from build123d import *

# Parameters (mm, degrees)
SZKIC2_W                    = 85
SZKIC2_H                    = 44.3
DODANIE_WYCI_GNI_CIE1_DEPTH = 1
SZKIC7_W                    = 85
SZKIC7_H                    = 1
DODANIE_WYCI_GNI_CIE2_DEPTH = 43
KONWERTUJ_START             = -42.5
KONWERTUJ_BRY_1_DEPTH       = 85
KONWERTUJ_BRY_1_2_DEPTH     = 85


# Read off the part's stored shape, not the designer's step: Konwertuj bryłę1
with BuildPart() as part:
    # Szkic2 → Dodanie-wyciągnięcie1 (new body)
    with BuildSketch(Plane(origin=(0, 0, 0), x_dir=(1, 0, 0), z_dir=(0, 1, 0))):
        Rectangle(SZKIC2_W, SZKIC2_H)
    extrude(amount=DODANIE_WYCI_GNI_CIE1_DEPTH)

    # Szkic7 → Dodanie-wyciągnięcie2 (add)
    with BuildSketch(Plane(origin=(0, 1, 0), x_dir=(1, 0, 0), z_dir=(0, 1, 0))):
        with Locations((0, 21.65)):
            Rectangle(SZKIC7_W, SZKIC7_H)
        with Locations((0, -21.65)):
            Rectangle(SZKIC7_W, SZKIC7_H)
    extrude(amount=DODANIE_WYCI_GNI_CIE2_DEPTH)

    # Konwertuj bryłę1 outline → Konwertuj bryłę1 (cut)
    with BuildSketch(Plane.YZ.offset(KONWERTUJ_START)):
        with BuildLine():
            ThreePointArc((2, -22.15), (0.585786438, -21.564213562), (0, -20.15))
            Line((0, -20.15), (0, -22.15))
            Line((0, -22.15), (2, -22.15))
        make_face()
        with BuildLine():
            ThreePointArc((0, 20.15), (0.585786438, 21.564213562), (2, 22.15))
            Line((2, 22.15), (0, 22.15))
            Line((0, 22.15), (0, 20.15))
        make_face()
    extrude(amount=KONWERTUJ_BRY_1_DEPTH, mode=Mode.SUBTRACT)

    # Konwertuj bry_1 2 outline → Konwertuj bry_1 2 (add)
    with BuildSketch(Plane.YZ.offset(KONWERTUJ_START)):
        with BuildLine():
            ThreePointArc((2, -21.15), (1.292893219, -20.857106781), (1, -20.15))
            Line((1, -20.15), (1, -21.15))
            Line((1, -21.15), (2, -21.15))
        make_face()
        with BuildLine():
            ThreePointArc((1, 20.15), (1.292893219, 20.857106781), (2, 21.15))
            Line((2, 21.15), (1, 21.15))
            Line((1, 21.15), (1, 20.15))
        make_face()
    extrude(amount=KONWERTUJ_BRY_1_2_DEPTH)


solid = part.part
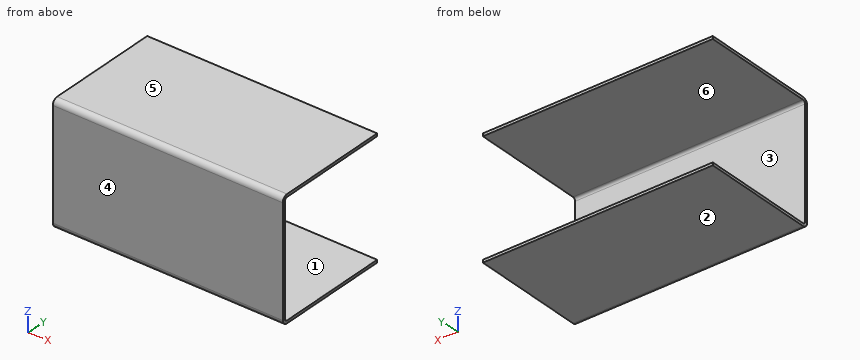
Model file for the job. Use its own axes, mm. Face numbers are marked on the shaded views. A direction names the side the tool comes from. Coordinates: 2 decimals unless noted, no trailing zeros. Write each loop counter-clockwise with the first axis right and the second up, starting at its lowest first coordinate (ties: lowest second). Pieces come first, ordered by that corner, then holes. Notation, with made-up numbers: (16, 51) -> (52, 51) arc R34 cw to (52, 82) -> close; hole circle Ø3 at (82, 14). An arc over 180 degrees is marked (long way). One line per item, written item: value. Start each with the question number.
1) Slice it at A-A on y = 22.5. Write the cut outline in (x, z).
2) Pull direction Z, two halves, no side cores. Call the marked faces 1, 2, 3 and 4: +Z half, -Z half, draft (parallel to the pull), parting line (faces both ways), or undercut.
3) Probe probe 1 along Z at (x, y) = (-37, 4.5); probe 2 along Y at (x, z) = (31, 14); probe 3 along Y at (x, z) = (22, 20.5). List the from-to ranges inside material, lowest first.
4) Slice it at C-C on z = -18. Write the cut outline in (x, y), then the cut area to 3 significant figures.
5) Which spindle directions (+Z, -Z, +X, -X, +Y, -Y) get a long thin tool onto all of the face, cutting with end or side? Do the marked faces 5 and 6. Say none if no direction does.
6) Flat gauge pins, fed straight in: pin 1 Ø3 at (x, z) = (24.5, 4) entering from -Y; pin 2 Ø12 at (x, z) = (18, 6.5) entering from +Y. Where does each tip first touch, or does it go through?
7) Slice it at B-B on x = -23.5. Write the cut outline in (y, z).
Answers follow:
1. outline: (-42.5, -22.15) -> (42.5, -22.15) -> (42.5, -21.15) -> (-42.5, -21.15) -> close; (-42.5, 21.15) -> (42.5, 21.15) -> (42.5, 22.15) -> (-42.5, 22.15) -> close
2. face 1: undercut
2. face 2: -Z half
2. face 3: undercut
2. face 4: draft
3. probe 1: -22.15 to -21.15, 21.15 to 22.15
3. probe 2: 0 to 1
3. probe 3: 0.03 to 1.06
4. outline: (-42.5, 0) -> (42.5, 0) -> (42.5, 1) -> (-42.5, 1) -> close
4. area: 85.0 mm2
5. face 5: +Z, +X, -X, +Y, -Y
5. face 6: +X, -X, +Y
6. pin 1: y = 0
6. pin 2: y = 1
7. outline: (0, -20.15) arc R2 ccw to (2, -22.15) -> (44, -22.15) -> (44, -21.15) -> (2, -21.15) arc R1 cw to (1, -20.15) -> (1, 20.15) arc R1 cw to (2, 21.15) -> (44, 21.15) -> (44, 22.15) -> (2, 22.15) arc R2 ccw to (0, 20.15) -> close
